from build123d import *

# Parameters (mm, degrees)
SKETCH001_W     = 38.319672
SKETCH001_H     = 14.959016
PAD_DEPTH       = 10
SKETCH_R        = 1.5
SKETCH_R_2      = 1.25
POCKET_DEPTH    = 10.001
SKETCH002_W     = 10.495989
SKETCH002_H     = 2.652832
POCKET001_DEPTH = 1
SKETCH003_R     = 3
POCKET002_DEPTH = 3


with BuildPart() as part:
    # Sketch001 → Pad (new body)
    with BuildSketch(Plane.XY):
        with Locations((9.016384, 0.102488)):
            Rectangle(SKETCH001_W, SKETCH001_H)
    extrude(amount=PAD_DEPTH)

    # Sketch → Pocket (cut, through all)
    with BuildSketch(Plane.XY):
        Circle(SKETCH_R)
        with Locations((18.341707, 0)):
            Circle(SKETCH_R_2)
    extrude(amount=POCKET_DEPTH, mode=Mode.SUBTRACT)

    # Sketch002 (on Face5 of Pocket) → Pocket001 (cut)
    with BuildSketch(Plane.XY.offset(10)):
        with Locations((8.792832, 3.447047)):
            Rectangle(SKETCH002_W, SKETCH002_H)
    extrude(amount=-POCKET001_DEPTH, mode=Mode.SUBTRACT)

    # Sketch003 (on Face5 of Pocket001) → Pocket002 (cut)
    with BuildSketch(Plane.XY.offset(10)):
        Circle(SKETCH003_R)
        with Locations((18.341707, 0)):
            Circle(SKETCH003_R)
    extrude(amount=-POCKET002_DEPTH, mode=Mode.SUBTRACT)


solid = part.part
Geometry: final body of the model. Coordinates: model frame, mm. A direction names the side the tool comes from. Coordinates: 2 decimals unless noted, no trailing zeros. Order: outer loops, then holes, each group sorted by start corner. A loop starts at its lowest first (then second) coordinate and runs counter-clockwise, first axis right, second up.
(1) Draft query along X for faces 3 (the face through (28.176, 0, 5)), 4 (the face through (9, 3, 9)), 5 (the face through (9, 0, 0)), 6 (the face through (19.496, -0.479, 3.451)). Return one class per face: pulls with the +X half, pulls with the -X half, needs draft (parallel to the pull), parting line crosses it, or undercut.
(2) Material intervals for probe 1 along X at (y, z) = (0, 3.5); probe 2 along X at (y, z) = (-1, 5.75); probe 3 along Y at (x, z) = (0, 4.75), sorted ascending.
(3) Section query B-B (y = 0). Return the cut outline in (x, z).
(4) Access query for faces 1 (the face through (-10.143, 0, 5)), 2 (the face through (1.3, -1.3, 7)). Directions: +Z, -Z, +X, -X, +Y, -Y. A direction counts if a zero-diameter tool reaches every point of the face in a straight line with its end or side. Return the directions, or none.
(5) Section query C-C (z = 3). Return the cut outline in (x, y), plus the area to 3 significant figures.
(6) Section query A-A (x = 0). Return the cut outline in (y, z).
(7) First-contact query: pin 1 (3 mm diameter, centred on x = -6, y = -5.5, fed in from -Z); pin 2 (5.5 mm diameter, centred on x = 0, y = 0, fed in from +Z). Flat tips, straight axial feed; report the tip coordinate or a pass-through.
(8) Section query D-D (z = 7.5). Return the cut outline in (x, y), plus the area to 3 significant figures.
Solution:
1. face 3: pulls with the +X half
1. face 4: undercut
1. face 5: needs draft
1. face 6: undercut
2. probe 1: x = -10.14 to -1.5, 1.5 to 17.09, 19.59 to 28.18
2. probe 2: x = -10.14 to -1.12, 1.12 to 17.59, 19.09 to 28.18
2. probe 3: y = -7.38 to -1.5, 1.5 to 7.58
3. outline: (-10.14, 0) - (-1.5, 0) - (-1.5, 7) - (-3, 7) - (-3, 10) - (-10.14, 10) - close; (1.5, 0) - (17.09, 0) - (17.09, 7) - (15.34, 7) - (15.34, 10) - (3, 10) - (3, 7) - (1.5, 7) - close; (19.59, 0) - (28.18, 0) - (28.18, 10) - (21.34, 10) - (21.34, 7) - (19.59, 7) - close
4. face 1: +Z, -Z, -X, +Y, -Y
4. face 2: +Z
5. outline: (-10.14, -7.38) - (28.18, -7.38) - (28.18, 7.58) - (-10.14, 7.58) - close; hole circle Ø3 at (0, 0); hole circle Ø2.5 at (18.34, 0)
5. area: 561 mm2
6. outline: (-7.38, 0) - (-1.5, 0) - (-1.5, 7) - (-3, 7) - (-3, 10) - (-7.38, 10) - close; (1.5, 0) - (7.58, 0) - (7.58, 10) - (3, 10) - (3, 7) - (1.5, 7) - close
7. pin 1: stops at z = 0
7. pin 2: stops at z = 7
8. outline: (-10.14, -7.38) - (28.18, -7.38) - (28.18, 7.58) - (-10.14, 7.58) - close; hole circle Ø6 at (0, 0); hole circle Ø6 at (18.34, 0)
8. area: 517 mm2
